```python
from build123d import *

# Parameters (mm, degrees)
SKETCH1_R               = 14
SKETCH1_R_2             = 1.25
BOSS_EXTRUDE1_DEPTH     = 7.75
SKETCH2_R               = 5
CUT_EXTRUDE1_DEPTH      = 1.9
SKETCH5_R               = 2.675
CUT_EXTRUDE3_DEPTH      = 3
SKETCH3_R               = 5.375
BOSS_EXTRUDE2_DEPTH     = 19
SKETCH4_R               = 1.25
CUT_EXTRUDE4_DEPTH      = 15
CUT_EXTRUDE4_DEPTH_BACK = 15


with BuildPart() as part:
    # Sketch1 → Boss-Extrude1 (new body)
    with BuildSketch(Plane(origin=(0, 0, 0), x_dir=(1, 0, 0), z_dir=(0, 1, 0))):
        Circle(SKETCH1_R)
        with Locations((-7.778174593, 7.778174593)):
            Circle(SKETCH1_R_2, mode=Mode.SUBTRACT)
        with Locations((0, 11)):
            Circle(SKETCH1_R_2, mode=Mode.SUBTRACT)
        with Locations((7.778174593, 7.778174593)):
            Circle(SKETCH1_R_2, mode=Mode.SUBTRACT)
        with Locations((11, 0)):
            Circle(SKETCH1_R_2, mode=Mode.SUBTRACT)
        with Locations((7.778174593, -7.778174593)):
            Circle(SKETCH1_R_2, mode=Mode.SUBTRACT)
        with Locations((0, -11)):
            Circle(SKETCH1_R_2, mode=Mode.SUBTRACT)
        with Locations((-11, 0)):
            Circle(SKETCH1_R_2, mode=Mode.SUBTRACT)
        with Locations((-7.778174593, -7.778174593)):
            Circle(SKETCH1_R_2, mode=Mode.SUBTRACT)
    extrude(amount=BOSS_EXTRUDE1_DEPTH)

    # Sketch2 → Cut-Extrude1 (cut)
    with BuildSketch(Plane(origin=(0, 7.75, 0), x_dir=(1, 0, 0), z_dir=(0, 1, 0))):
        Circle(SKETCH2_R)
    extrude(amount=-CUT_EXTRUDE1_DEPTH, mode=Mode.SUBTRACT)

    # Sketch5 → Cut-Extrude3 (cut)
    with BuildSketch(Plane(origin=(0, 5.85, 0), x_dir=(1, 0, 0), z_dir=(0, 1, 0))):
        Circle(SKETCH5_R)
    extrude(amount=-CUT_EXTRUDE3_DEPTH, mode=Mode.SUBTRACT)

    # Sketch3 → Boss-Extrude2 (add)
    with BuildSketch(Plane.XZ):
        Circle(SKETCH3_R)
    extrude(amount=BOSS_EXTRUDE2_DEPTH)

    # Sketch4 → Cut-Extrude4 (cut, two sides)
    with BuildSketch(Plane.XY) as cut_extrude4_sk:
        with Locations((0, -7.5)):
            Circle(SKETCH4_R)
    extrude(amount=CUT_EXTRUDE4_DEPTH, mode=Mode.SUBTRACT)
    extrude(cut_extrude4_sk.sketch, amount=-CUT_EXTRUDE4_DEPTH_BACK, mode=Mode.SUBTRACT)


solid = part.part
```
Build history of the part. All positions in model axes, mm. A direction names the side the tool comes from. Round coordinates to 2 decimals unless told otherwise and drop trailing zeros. Write each loop counter-clockwise with the first axis right and the second up, starting at its lowest first coordinate (ties: lowest second). Pieces come first, ordered by that corner, then holes. Notation, with made-up numbers: (-10, 47.5) - (15, 47.5) arc R20 ccw to (15, 59.5) - close; hole circle Ø10 at (-1.75, 55). An arc over 180 degrees is marked (long way). Answer as CSV lines item,"result".
Q1. Cut at B-B (z = 11.5). Write the cut outline in (x, y).
Report:
outline,"(-7.98, 0) - (-1.15, 0) - (-1.15, 7.75) - (-7.98, 7.75) - close; (1.15, 0) - (7.98, 0) - (7.98, 7.75) - (1.15, 7.75) - close"
Q2. Drop flat-ended pins along their axis: pin 1 (8 mm diameter, centred on x = -2.5, z = -2, fed in from +Y); pin 2 (4 mm diameter, centred on x = 0, y = -7.5, fed in from -Z) (3 decimals); pin 3 (2 mm diameter, centred on x = 0, y = -7.5, fed in from -Z); pin 4 (6 mm diameter, centred on x = -1, z = -0.5, fed in from +Y). Give the stop position or say it passes through.
Report:
pin 1,"stops at y = 7.75"
pin 2,"stops at z = -5.375"
pin 3,"passes through"
pin 4,"stops at y = 5.85"
Q3. Cut at A-A (x = -11). Write the cut outline in (y, z), and give its area (3 significant figures).
Report:
outline,"(0, -8.66) - (7.75, -8.66) - (7.75, -1.25) - (0, -1.25) - close; (0, 1.25) - (7.75, 1.25) - (7.75, 8.66) - (0, 8.66) - close"
area,"115 mm^2"
Q4. Pull direction X, two halves, no side cores. Call faces 4 (the cylindrical face through (-0.16, 3.82, -12.24)), 5 (the flat face through (0, 7.75, 6)), 6 (the cylindrical face through (12.932, 3.821, 5.362)): +X half, -X half, draft (parallel to the pull), parting line (faces both ways), or undercut.
Report:
face 4,"undercut"
face 5,"draft"
face 6,"parting line"
Q5. Tool access for faces 1 (the flat face through (0, 0, 6)), 2 (the cylindrical face through (9.75, 3.82, -0.05)), 3 (the cylindrical face through (-0.58, 4.37, 2.61)): list every direction of +Z, -Z, +X, -X, +Y, -Y with a clear straight run to the whole face (end or side of a thin tool).
Report:
face 1,"-Y"
face 2,"+Y, -Y"
face 3,"+Y"
Q6. Drill centre lines: probe 1 along X at (y, z) = (3.7, 0) (3 decimals); probe 2 along Y at (x, z) = (0, -2.3); probe 3 along Y at (x, z) = (0, 2.95). Where is each one in solid material? Low to high. Write a range as [from, to].
Report:
probe 1,"x = [-14, -12.25], [-9.75, -2.675], [2.675, 9.75], [12.25, 14]"
probe 2,"y = [-19, -8.75], [-6.25, 2.85]"
probe 3,"y = [-19, -8.75], [-6.25, 5.85]"
Q7. Cut at C-C (x = -7.75). Write the cut outline in (y, z), and give its area (3 significant figures).
Report:
outline,"(0, -11.66) - (7.75, -11.66) - (7.75, -9.03) - (0, -9.03) - close; (0, -6.53) - (7.75, -6.53) - (7.75, 6.53) - (0, 6.53) - close; (0, 9.03) - (7.75, 9.03) - (7.75, 11.66) - (0, 11.66) - close"
area,"142 mm^2"
Q8. Cut at D-D (y = -7.5). Write the cut outline in (x, z) (3 decimals).
Report:
outline,"(-1.25, -5.228) - (-1.25, 5.228) arc R5.375 ccw to start; (1.25, -5.228) arc R5.375 ccw to (1.25, 5.228) - close"
